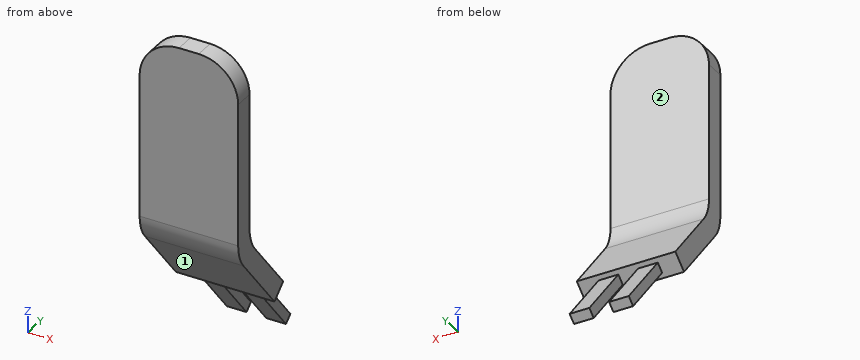
from build123d import *

# Parameters (mm, degrees)
BOSS_EXTRUDE1_DEPTH = 2.5
FILLET1_R           = 1
FILLET2_R           = 1
SKETCH3_W           = 0.5
SKETCH3_H           = 0.25
BOSS_EXTRUDE2_DEPTH = 2


with BuildPart() as part:
    # Sketch1 → Boss-Extrude1 (new body)
    with BuildSketch(Plane(origin=(0, 0, 0), x_dir=(0, 0, -1), z_dir=(1, 0, 0))):
        Polygon((0, 0), (5, 0), (6.924233249, 1.596034587), (6.605026331, 1.980881237), (4.819625854, 0.5), (0, 0.5), align=None)
    extrude(amount=BOSS_EXTRUDE1_DEPTH)

    # Fillet1
    fillet1_edges = [part.edges().sort_by_distance(p)[0] for p in [
        (2.5, 0.25, 0),
        (0, 0.25, 0),
    ]]
    fillet(fillet1_edges, radius=FILLET1_R)

    # Fillet2
    fillet2_edges = [part.edges().sort_by_distance(p)[0] for p in [
        (1.25, 0.5, -4.819625854),
        (1.25, 0, -5),
    ]]
    fillet(fillet2_edges, radius=FILLET2_R)

    # Sketch3 → Boss-Extrude2 (add)
    with BuildSketch(Plane(origin=(0, 4.052948843, -4.886372126), x_dir=(-1, 0, 0), z_dir=(0, 0.6384138349157521, -0.7696932995603917))):
        with Locations((-1.75, -2.942069175)):
            Rectangle(SKETCH3_W, SKETCH3_H)
        with Locations((-0.75, -2.942069175)):
            Rectangle(SKETCH3_W, SKETCH3_H)
    extrude(amount=BOSS_EXTRUDE2_DEPTH)


solid = part.part
Part model, mm, in its own coordinate system. Face numbers are marked on the shaded views. A direction names the side the tool comes from. Give positions to 0.01 mm unless a question says otherwise; leave off trailing zeros. Loops run counter-clockwise (first coordinate to the right, second up) from the corner with the lowest first, then second, coordinate; pieces in that order, holes last. Notation, with made-up numbers: (3, 4) -> (17, 4) arc R19 ccw to (17, 36) -> close; hole circle Ø11 at (57.25, 8). An arc over 180 degrees is marked (long way). Write each question's results on one line, items separated by ' | '. Start each with the question number.
Q1. Band-saw the part on B-B on y = 2.6. List the corners of the cut face in (x, z), plus the area to 3 significant figures.
Q2. Band-saw the part on C-C on x = 2.2. List the corners of the cut face in (y, z), plus the area to 3 significant figures.
Q3. Which spindle directions (+Z, -Z, +X, -X, +Y, -Y) get a long thin tool onto all of the face, cutting with end or side? Do the marked faces 1 and 2. Say none if no direction does.
Q4. Pin check, flat tips, straight feed: P1, Ø0.8, axis at x = 2, z = -2, coming from the +Y side; P2, Ø1.2, axis at y = 2.5, z = -7.5, coming from the -X side; P3, Ø0.7, axis at y = 2.5, z = -7, coming from the +X side. Stop position of each tip, or through.
Q5. Wall check: L1, parallel to Y at x = 1.4, z = -3.5; L2, parallel to Z at x = 0.7, y = 1.05; L3, parallel to Z at x = 1.55, y = 2.4. Give the ranges that are in metal, low to high.
Q6. Band-saw the part on A-A on z = -7.25. List the corners of the cut face in (x, y), plus the area to 3 significant figures.
Q7. Band-saw the part on D-D on z = -3. List the corners of the cut face in (x, y).
Results are:
1) outline: (0.5, -7.94) -> (1, -7.94) -> (1, -7.55) -> (0.5, -7.55) -> close; (1.5, -7.94) -> (2, -7.94) -> (2, -7.55) -> (1.5, -7.55) -> close | area: 0.392 mm²
2) outline: (0, -4.64) arc R1 ccw to (0.23, -5.28) -> (1.6, -6.92) -> (1.98, -6.61) -> (0.73, -5.1) arc R1 cw to (0.5, -4.46) -> (0.5, -0.29) -> (0, -0.29) -> close | area: 3.52 mm²
3) face 1: -Z, +X, -X, -Y | face 2: +Z, +X, -X, +Y
4) P1: stops at y = 0.5 | P2: stops at x = 0.5 | P3: stops at x = 2
5) L1: y = 0 to 0.5 | L2: z = -6.27 to -5.48 | L3: z = -7.7 to -7.31
6) outline: (0.5, 2.03) -> (1, 2.03) -> (1, 2.35) -> (0.5, 2.35) -> close; (1.5, 2.03) -> (2, 2.03) -> (2, 2.35) -> (1.5, 2.35) -> close | area: 0.325 mm²
7) outline: (0, 0) -> (2.5, 0) -> (2.5, 0.5) -> (0, 0.5) -> close
